from build123d import *

# Parameters (mm, degrees)
SKETCH1_R      = 0.5207
EXTRUDE1_DEPTH = 0.3175
FILLET1_R      = 0.7874


with BuildPart() as part:
    # Sketch1 → Extrude1 (new body, symmetric)
    with BuildSketch(Plane(origin=(0, 0, 0), x_dir=(0, 0, -1), z_dir=(1, 0, 0))):
        with BuildLine():
            Line((-0.389621032, 4.453388778), (-0.584431549, 6.680083168))
            Line((-0.584431549, 6.680083168), (-2.25445234, 6.53397528))
            Line((-2.25445234, 6.53397528), (-2.87534029, 4.386740502))
            ThreePointArc((-2.87534029, 4.386740502), (0, -5.7404), (2.87534029, 4.386740502))
            Line((2.87534029, 4.386740502), (2.25445234, 6.53397528))
            Line((2.25445234, 6.53397528), (0.584431549, 6.680083168))
            Line((0.584431549, 6.680083168), (0.389621032, 4.453388778))
            ThreePointArc((0.389621032, 4.453388778), (0, -4.4704), (-0.389621032, 4.453388778))
        make_face()
        with Locations((-1.322036686, 5.493682029)):
            Circle(SKETCH1_R, mode=Mode.SUBTRACT)
        with Locations((1.322036686, 5.493682029)):
            Circle(SKETCH1_R, mode=Mode.SUBTRACT)
    extrude(amount=EXTRUDE1_DEPTH, both=True)

    # Fillet1
    fillet1_edges = [part.edges().sort_by_distance(p)[0] for p in [
        (0, 6.53397528, -2.25445234),
        (0, 4.386740502, -2.87534029),
        (0, 4.386740502, 2.87534029),
        (0, 6.53397528, 2.25445234),
    ]]
    fillet(fillet1_edges, radius=FILLET1_R)


solid = part.part
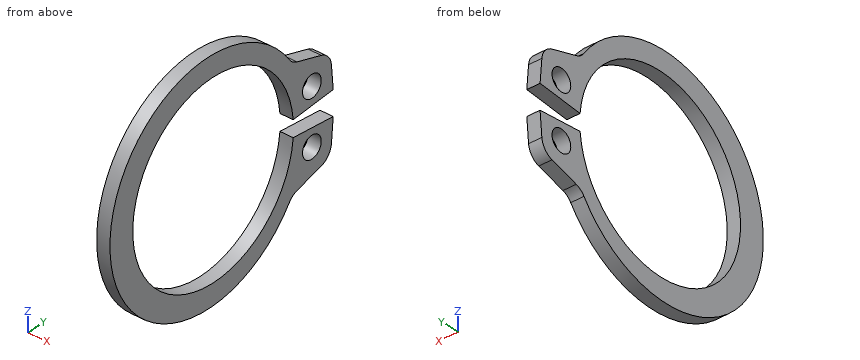
Design review of the part built by this model. Coordinates are the model's own, in mm. Round coordinates to 2 decimals unless told otherwise and drop trailing zeros. Write each loop counter-clockwise with the first axis right and the second up, starting at its lowest first coordinate (ties: lowest second). Pieces come first, ordered by that corner, then holes. Notation, with made-up numbers: (84.5, 21.5) - (118.5, 21.5) arc R17 ccw to (118.5, 25.5) - close; hole circle Ø7 at (55.5, 29). An arc over 180 degrees is marked (long way). Use a Markdown table: item, result. Add a question column.
1. We need section B-B (x = -0.1). State the section outline as (y, z) points.
2. We need section C-C (z = 0). State the section outline as (x, y) points.
3. We need section A-A (y = 2.75). State the section outline as (x, z) points, then the cut area to 3 significant figures.
4. We need section D-D (y = 0). State the section outline as (x, z) points.
5. Wall thickness on probe 1 along Z at (x, y) = (0.15, 5.25); probe 2 along Z at (x, y) = (0.2, 5.75); probe 3 along Z at (x, y) = (-0.15, -0.5): over which ranges is each line inside the solid? List them lowest first.
Output:
| question | item | result |
|---|---|---|
| 1 | outline | (4.24, -3.1) arc R0.79 cw to (4.67, -2.79) - (6.02, -2.4) arc R0.79 ccw to (6.58, -1.72) - (6.68, -0.58) - (4.45, -0.39) arc R4.47 cw (long way) to (4.45, 0.39) - (6.68, 0.58) - (6.58, 1.72) arc R0.79 ccw to (6.02, 2.4) - (4.67, 2.79) arc R0.79 cw to (4.24, 3.1) arc R5.47 ccw (long way) to start; hole circle Ø1.04 at (5.49, -1.32); hole circle Ø1.04 at (5.49, 1.32) |
| 2 | outline | (-0.32, -5.74) - (0.32, -5.74) - (0.32, -4.47) - (-0.32, -4.47) - close |
| 3 | outline | (-0.32, -4.56) - (0.32, -4.56) - (0.32, -3.52) - (-0.32, -3.52) - close; (-0.32, 3.52) - (0.32, 3.52) - (0.32, 4.56) - (-0.32, 4.56) - close |
| 3 | area | 1.32 mm2 |
| 4 | outline | (-0.32, -5.47) - (0.32, -5.47) - (0.32, -4.47) - (-0.32, -4.47) - close; (-0.32, 4.47) - (0.32, 4.47) - (0.32, 5.47) - (-0.32, 5.47) - close |
| 5 | probe 1 | z = -2.63 to -1.78, -0.86 to -0.46, 0.46 to 0.86, 1.78 to 2.63 |
| 5 | probe 2 | z = -2.48 to -1.78, -0.87 to -0.5, 0.5 to 0.87, 1.78 to 2.48 |
| 5 | probe 3 | z = -5.47 to -4.44, 4.44 to 5.47 |
